from build123d import *

# Parameters (mm, degrees)
F0_R     = 7.9248
F1_DEPTH = 5.08
F2_R     = 1.27
F3_R     = 3.175
F4_DEPTH = 25.4


with BuildPart() as f1:
    # F0 (on Front) → F1 (new body)
    with BuildSketch(Plane.XZ):
        Polygon((-25.72123, 13.428098), (-44.45, 0), (-25.72123, -13.428098), (25.72123, -13.428098), (44.45, 0), (25.72123, 13.428098), align=None)
        Circle(F0_R, mode=Mode.SUBTRACT)
    extrude(amount=F1_DEPTH)

    # F2
    f2_edges = [f1.edges().sort_by_distance(p)[0] for p in [
        (44.45, -2.54, 0),
        (-44.45, -2.54, 0),
    ]]
    fillet(f2_edges, radius=F2_R)

    # F3 (on face) → F4 (cut)
    with BuildSketch(Plane.XZ.offset(5.08)):
        with Locations((-25.625831, 7.596325)):
            Circle(F3_R)
        with Locations((-25.625831, 0)):
            Circle(F3_R)
        with Locations((-25.625831, -7.464381)):
            Circle(F3_R)
        with Locations((-34.600362, 0)):
            Circle(F3_R)
        with Locations((25.625831, 0)):
            Circle(F3_R)
        with Locations((25.625831, 7.596325)):
            Circle(F3_R)
        with Locations((34.600362, 0)):
            Circle(F3_R)
        with Locations((25.625831, -7.464381)):
            Circle(F3_R)
    extrude(amount=-F4_DEPTH, mode=Mode.SUBTRACT)


solid = f1.part
The listing builds one solid part. Answer for the finished solid, in the listing's coordinates (mm). Coordinates: 2 decimals unless noted, no trailing zeros. Write each loop counter-clockwise with the first axis right and the second up, starting at its lowest first coordinate (ties: lowest second). Pieces come first, ordered by that corner, then holes. Notation, with made-up numbers: M 86,30.25 L 99,30.25 A18 cw 99,49.25 Z; hole C -38,57.5 d2. An arc over 180 degrees is marked long. Use one line per item in the form item = value.
Item 1: Find section D-D, the plane x = 33.5. Give the vertices of the cut face in (y, z), plus the area to 3 significant figures.
Model answer:
outline = M -5.08,-7.85 L 0,-7.85 L 0,-2.98 L -5.08,-2.98 Z; M -5.08,2.98 L 0,2.98 L 0,7.85 L -5.08,7.85 Z
area = 49.5 mm2
Item 2: Find the intervals of material crossed by probe 1 along X at (y, z) = (-4.05, -4.75); probe 2 along Z at (x, y) = (0, -3.35); probe 3 along X at (y, z) = (-3.45, -1.25), in increasing order.
Model answer:
probe_1 = -37.82 to -27.27, -23.98 to -6.34, 6.34 to 23.98, 27.27 to 37.82
probe_2 = -13.43 to -7.92, 7.92 to 13.43
probe_3 = -42.71 to -37.52, -31.68 to -28.54, -22.71 to -7.83, 7.83 to 22.71, 28.54 to 31.68, 37.52 to 42.71
Item 3: Find section C-C, the plane y = -2.25. Give the number of separate pieces and of enclosed holes in the cut face, plus the area to 3 significant figures.
Model answer:
separate_pieces = 1
enclosed_holes = 9
area = 1,430 mm2
Item 4: Find section A-A, the plane z = 0. Give the vertices of the cut face in (x, y).
Model answer:
outline = M -43.54,-5.08 L -37.78,-5.08 L -37.78,0 L -43.54,0 Z; M -31.43,-5.08 L -28.8,-5.08 L -28.8,0 L -31.43,0 Z; M -22.45,-5.08 L -7.92,-5.08 L -7.92,0 L -22.45,0 Z; M 7.92,-5.08 L 22.45,-5.08 L 22.45,0 L 7.92,0 Z; M 28.8,-5.08 L 31.43,-5.08 L 31.43,0 L 28.8,0 Z; M 37.78,-5.08 L 43.54,-5.08 L 43.54,0 L 37.78,0 Z
Item 5: The mould has two halves that part along Z. Classify faces 1 (the face through (-10, -5.08, 0)), 2 (the face through (-34.49, -2.5, -7.14)), 3 (the face through (-1.032, -2.504, 7.857)), 4 (the face through (34.49, -2.5, 7.14)): released by +Z, released by -Z, zero draft, split by the parting line, or undercut.
Model answer:
face_1 = zero draft
face_2 = released by -Z
face_3 = undercut
face_4 = released by +Z
Item 6: Find section B-B, the plane x = 0. Give the vertices of the cut face in (y, z), plus the area to 3 significant figures.
Model answer:
outline = M -5.08,-13.43 L 0,-13.43 L 0,-7.92 L -5.08,-7.92 Z; M -5.08,7.92 L 0,7.92 L 0,13.43 L -5.08,13.43 Z
area = 55.9 mm2
